```python
from build123d import *

# Parameters (mm, degrees)
F0_R       = 29.75
F1_DEPTH   = 2
F3_DEPTH   = 30
F4_SIZE2   = 19.0811366877
F4_SIZE    = 1
F5_SIZE2   = 1.0013554388
F5_SIZE    = 19.107
F5_2_SIZE2 = 1.0013554388
F5_2_SIZE  = 19.107
F6_SIZE    = 1.5


with BuildPart() as f1:
    # F0 (on Top) → F1 (new body)
    with BuildSketch(Plane.XY):
        Circle(F0_R)
    extrude(amount=F1_DEPTH)

    # F2 (on face) → F3 (join)
    with BuildSketch(Plane.XY.offset(2)):
        Polygon((10.3176952883, -12.6805032999), (-16.307790299, 1.1427928787), (-17.614022031, -1.3731811483), (-14.2932211873, -13.4240019402), (-2.7555107662, -19.4140969509), (9.0114635564, -15.1964773269), align=None)
        Polygon((-8.5677054632, 14.9660890572), (-9.8739371952, 12.4501150302), (16.7515483921, -1.3731811483), (18.0577801241, 1.1427928787), (14.7369792805, 13.1936136705), (3.1992688593, 19.1837086812), align=None)
    extrude(amount=F3_DEPTH)

    # F4
    f4_edges = [f1.edges().sort_by_distance(p)[0] for p in [
        (3.438806, 5.538467, 32),
        (8.968124, 16.188661, 32),
    ]]
    f4_side = f1.faces().sort_by_distance((5.828725, 10.141766, 32))[0]
    chamfer(f4_edges, length=F4_SIZE, length2=F4_SIZE2, reference=f4_side)

    # F5
    f5_edges = [f1.edges().sort_by_distance(p)[0] for p in [
        (-2.995048, -5.768855, 32),
    ]]
    f5_side = f1.faces().sort_by_distance((-2.995048, -5.768855, 17))[0]
    chamfer(f5_edges, length=F5_SIZE, length2=F5_SIZE2, reference=f5_side)

    # F5#2
    f5_2_edges = [f1.edges().sort_by_distance(p)[0] for p in [
        (-8.524366, -16.419049, 32),
    ]]
    f5_2_side = f1.faces().sort_by_distance((-8.524366, -16.419049, 17))[0]
    chamfer(f5_2_edges, length=F5_2_SIZE, length2=F5_2_SIZE2, reference=f5_2_side)

    # F6
    f6_edges = [f1.edges().sort_by_distance(p)[0] for p in [
        (-29.75, 0, 0),
    ]]
    chamfer(f6_edges, length=F6_SIZE)


solid = f1.part
```
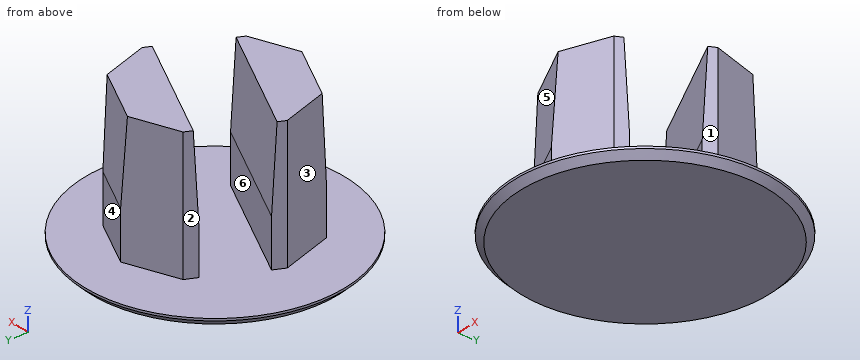
Geometry check sheet. Reference: the model listing, model coordinates, mm. Face numbers are marked on the shaded views. A direction names the side the tool comes from. Round coordinates to 2 decimals unless told otherwise and drop trailing zeros. Loops run counter-clockwise (first coordinate to the right, second up) from the corner with the lowest first, then second, coordinate; pieces in that order, holes last. Notation, with made-up numbers: M 25,32.5 L 65,32.5 A30 ccw 65,67.5 Z; hole C 40,-29 d2. An arc over 180 degrees is marked long. Return JSON: item names as keys, results as strings. Group by question number.
(1) Mould release check, pull along Y, two halves, no side actions. Record for the marked faces 4, 5 and 6: pulls with the +Y half, pulls with the -Y half, needs draft (parallel to the pull), parting line crosses it, or undercut.
(2) Section check A-A, the plane z = 6. Enter the section's corners in (x, y), and give its area (3 significant figures).
(3) Section check B-B, the plane x = 0. Enter the section's corners in (y, z).
(4) Section check C-C, the plane z = 20. Enter the section's corners in (x, y), and give its area (3 significant figures).
(5) Go/stop test with flat-tipped pins: pin 1 (2 mm diameter, centred on x = -14.5, y = 19.5, fed in from +Z); pin 2 (4 mm diameter, centred on x = -7.5, z = 27.5, fed in from +Y); pin 3 (5 mm diameter, centred on y = 8, z = 17.5, fed in from -X). Record where each tip stops, or that it passes through.
(6) Scan lines: line 1 along Z through (x, y) = (16, -11); line 2 along Y through (x, z) = (-7, 21.5); line 3 along Y through (x, z) = (7, 2.5). Record each from-to range of solid material in increasing order. Write a range as [from, to].
(7) Set-up check for the marked faces 1, 2 and 3: record each of +Z, -Z, +X, -X, +Y, -Y from which the full face is reachable in a straight line by a thin tool's end or side.
Data:
{
 "1": {"face 4": "pulls with the +Y half", "face 5": "pulls with the -Y half", "face 6": "undercut"},
 "2": {"outline": "M -17.61,-1.37 L -14.29,-13.42 L -2.76,-19.41 L 9.01,-15.2 L 10.32,-12.68 L -16.31,1.14 Z; M -9.87,12.45 L 16.75,-1.37 L 18.06,1.14 L 14.74,13.19 L 3.2,19.18 L -8.57,14.97 Z", "area": "564 mm²"},
 "3": {"outline": "M -29.75,1.5 L -28.25,0 L 28.25,0 L 29.75,1.5 L 29.75,2 L 18.04,2 L 18.04,32 L 8.45,32 L 7.32,12.92 L 7.32,2 L -7.32,2 L -7.32,12.89 L -8.45,32 L -18.43,32 L -18.43,2 L -29.75,2 Z"},
 "4": {"outline": "M -17.61,-1.37 L -14.43,-12.93 L -2.28,-19.24 L 9.01,-15.2 L 10.15,-13.01 L -16.48,0.81 Z; M -9.7,12.78 L 16.92,-1.04 L 18.06,1.14 L 14.87,12.71 L 2.72,19.01 L -8.57,14.97 Z", "area": "532 mm²"},
 "5": {"pin 1": "z = 2", "pin 2": "y = 16.07", "pin 3": "x = -5.61"},
 "6": {"line 1": "[0, 2]", "line 2": "[-16.7, -4.2], [11.46, 15.53]", "line 3": "[-15.92, -10.96], [3.69, 17.21]"},
 "7": {"face 1": "+Z, +X, -Y", "face 2": "+Z, -X, +Y", "face 3": "+Z, -X, -Y"}
}
